```python
from build123d import *

# Parameters (mm, degrees)
EXTRUDE_1_DEPTH     = 1383.55
SKETCH_2_W          = 6.397518836
SKETCH_2_H          = 13.287823591
CUT_EXTRUDE_1_DEPTH = 22.764865627


with BuildPart() as part:
    # Эскиз1 → Бобышка-Вытянуть1 (new body)
    with BuildSketch(Plane(origin=(0, 0, 0), x_dir=(1, 0, 0), z_dir=(0, 1, 0))):
        Polygon((-11.764865627, 15), (10, 15), (10, 1.25), (6, 1.25), (6, -1.25), (10, -1.25), (10, -15), (-11.764865627, -15), align=None)
    extrude(amount=EXTRUDE_1_DEPTH)

    # Эскиз2 → Вырез-Вытянуть1 (cut, through all)
    with BuildSketch(Plane.ZY.offset(11.764865627)):
        with Locations((0, 6.643911796)):
            Rectangle(SKETCH_2_W, SKETCH_2_H)
        with Locations((0, 1376.906088205)):
            Rectangle(SKETCH_2_W, SKETCH_2_H)
    extrude(amount=-CUT_EXTRUDE_1_DEPTH, mode=Mode.SUBTRACT)


solid = part.part
```
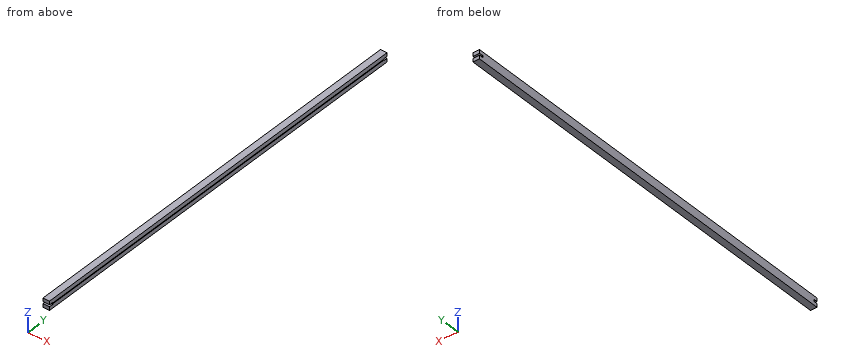
Geometry check sheet. Reference: the model listing, model coordinates, mm. Round coordinates to 2 decimals unless told otherwise and drop trailing zeros. Loops run counter-clockwise (first coordinate to the right, second up) from the corner with the lowest first, then second, coordinate; pieces in that order, holes last. Notation, with made-up numbers: (34, 18.25) - (75, 18.25) arc R21 ccw to (75, 23.25) - close; hole circle Ø8 at (35.5, 26.5). An arc over 180 degrees is marked (long way). Use a Markdown table: item, result.
Q1. Go/stop test with flat-tipped pins: P1, Ø3, axis at x = -5, z = 0, coming from the -Y side; P2, Ø0.8, axis at y = 658, z = 0, coming from the +X side; P3, Ø3, axis at x = -2.5, z = 1.5, coming from the +Y side. Record where each tip stops, or that it passes through.
Solutions:
| item | result |
|---|---|
| P1 | stops at y = 13.29 |
| P2 | stops at x = 6 |
| P3 | stops at y = 1370.26 |
Q2. Cross-section at A-A on y = 1024.5. Record the cut outline in (x, z), plus the area to 3 significant figures.
Solutions:
| item | result |
|---|---|
| outline | (-11.76, -15) - (10, -15) - (10, -1.25) - (6, -1.25) - (6, 1.25) - (10, 1.25) - (10, 15) - (-11.76, 15) - close |
| area | 643 mm2 |
Q3. Material ranges on line 1 (Z direction, x = 7.5, y = 921); line 2 (X direction, y = 769, z = -0.75), recorded low to high.
Solutions:
| item | result |
|---|---|
| line 1 | z = -15 to -1.25, 1.25 to 15 |
| line 2 | x = -11.76 to 6 |
